from build123d import *

# Parameters (mm, degrees)
F1_DEPTH = 5


with BuildPart() as f1:
    # F0 (on Top) → F1 (new body)
    with BuildSketch(Plane.XY):
        with BuildLine():
            ThreePointArc((379.525959, 223.226488), (379.643478, 223.344661), (379.760338, 223.463485))
            Line((379.760338, 223.463485), (379.428555, 223.323892))
            Line((379.428555, 223.323892), (379.525959, 223.226488))
        make_face()
        with BuildLine():
            ThreePointArc((379.760338, 223.463485), (386.092492, 233.113339), (388.312756, 244.439691))
            ThreePointArc((388.312756, 244.439691), (388.310904, 244.773005), (388.305349, 245.106277))
            ThreePointArc((388.305349, 245.106277), (330.470527, 255.611544), (379.525959, 223.226488))
            Line((379.525959, 223.226488), (379.428555, 223.323892))
            Line((379.428555, 223.323892), (379.760338, 223.463485))
        make_face()
        Polygon((337.001699, 235.473338), (337.001699, 253.128634), (343.146089, 253.156912), (343.146089, 250.818692), (343.146089, 250.623444), (343.146089, 235.485236), align=None, mode=Mode.SUBTRACT)
        Polygon((349.594001, 229.606358), (367.031511, 229.606358), (367.001699, 223.128634), (349.623813, 223.128634), align=None, mode=Mode.SUBTRACT)
        Polygon((373.146089, 235.543326), (373.146089, 253.294979), (379.428555, 253.323892), (379.428555, 235.555491), align=None, mode=Mode.SUBTRACT)
        Polygon((360.944925, 246.99601), (360.921156, 241.831291), (360.938548, 241.813899), (360.921076, 241.813899), (355.686963, 241.813899), (355.686963, 246.989038), (355.686963, 247.007774), (355.706094, 246.989064), (360.868974, 246.99591), (360.945276, 247.072211), align=None, mode=Mode.SUBTRACT)
        Polygon((367.168043, 259.273024), (349.457468, 259.273024), (349.428555, 265.555491), (367.196957, 265.555491), align=None, mode=Mode.SUBTRACT)
    extrude(amount=F1_DEPTH)


solid = f1.part
Design review of the part built by this model. Coordinates are the model's own, in mm. A direction names the side the tool comes from. Round coordinates to 2 decimals unless told otherwise and drop trailing zeros. Loops run counter-clockwise (first coordinate to the right, second up) from the corner with the lowest first, then second, coordinate; pieces in that order, holes last. Notation, with made-up numbers: M 51.5,84.5 L 88.5,84.5 A20 ccw 88.5,116.5 Z; hole C 27,-38 d3. An arc over 180 degrees is marked long. Answer as a JSON object with one key per item and string values.
Item 1: We need section C-C on z = 1. State how many separate pieces and enclosed holes the cut face has, and give its area (3 significant figures).
Answer sheet:
{"separate pieces": "1", "enclosed holes": "5", "area": "2,360 mm^2"}
Item 2: We need section D-D on y = 252. Give the boundary of the cut face in (x, z).
Answer sheet:
{"outline": "M 329.28,0 L 337,0 L 337,5 L 329.28,5 Z; M 343.15,0 L 373.15,0 L 373.15,5 L 343.15,5 Z; M 379.43,0 L 387.34,0 L 387.34,5 L 379.43,5 Z"}
Item 3: We need section B-B on y = 224.5. Give the boundary of the cut face in (x, z).
Answer sheet:
{"outline": "M 335.9,0 L 349.62,0 L 349.62,5 L 335.9,5 Z; M 367.01,0 L 380.73,0 L 380.73,5 L 367.01,5 Z"}
Item 4: Clearance check with flat-ended pins moving along their axes: P1, Ø1, axis at y = 257.5, z = 3.5, coming from the +X side; P2, Ø1.5, axis at y = 247, z = 3, coming from the +X side; P3, Ø4, axis at x = 371.5, y = 233.5, coming from the -Z side; P4, Ø1.5, axis at y = 243, z = 1.5, coming from the -X side. State where each tip first meets the part, or that it passes through.
Answer sheet:
{"P1": "stops at x = 385.56", "P2": "stops at x = 388.26", "P3": "stops at z = 0", "P4": "stops at x = 328.32"}
Item 5: Machinability: for faces 4 (the flat face through (358, 238, 5)), 5 (the flat face through (355.687, 244, 2)), which of the approach directions +Z, -Z, +X, -X, +Y, -Y give a long, thin tool a straight path to every point of the face, cutting with its end or side? Answer none if there is none.
Answer sheet:
{"face 4": "+Z, +X, -X, +Y, -Y", "face 5": "+Z, -Z"}
Item 6: We need section A-A on x = 376.5. Give the boundary of the cut face in (y, z), and give its area (3 significant figures).
Answer sheet:
{"outline": "M 220.58,0 L 235.55,0 L 235.55,5 L 220.58,5 Z; M 253.31,0 L 268.3,0 L 268.3,5 L 253.31,5 Z", "area": "150 mm^2"}
Item 7: Wall thickness on L1, parallel to X at y = 245, z = 3.75; L2, parallel to Y at x = 359, z = 4.45; L3, parallel to Y at x = 362, z = 1.15: over which ranges is each line inside the solid? List them lowest first. Write a range as from..to.
Answer sheet:
{"L1": "x = 328.32..337, 343.15..355.69, 360.94..373.15, 379.43..388.31", "L2": "y = 214.45..223.13, 229.61..241.81, 246.99..259.27, 265.56..274.43", "L3": "y = 214.67..223.13, 229.61..259.27, 265.56..274.21"}
Item 8: The part is to be moulded in two halves that separate along Y. For faces 1 (the cylindrical face through (330.92, 256.67, 2.46)), 2 (the flat face through (337.002, 244, 2)), 3 (the cylindrical face through (386.03, 232.96, 2.46)), say which applies: pulls with the +Y half, pulls with the -Y half, needs draft (parallel to the pull), parting line crosses it, or undercut.
Answer sheet:
{"face 1": "parting line crosses it", "face 2": "undercut", "face 3": "pulls with the -Y half"}
